The listing builds one solid part. Answer for the finished solid, in the listing's coordinates (mm). A direction names the side the tool comes from. Give positions to 0.01 mm unless a question says otherwise; leave off trailing zeros. Loops run counter-clockwise (first coordinate to the right, second up) from the corner with the lowest first, then second, coordinate; pieces in that order, holes last. Notation, with made-up numbers: M 61.5,-17 L 99.5,-17 A32 ccw 99.5,9 Z; hole C -21,-26 d5. An arc over 180 degrees is marked long. Use one line per item in the form item = value. Start each with the question number.
1. Each of these flat-tipped pins is pushed along its axis until it touches: pin 1 Ø4 at (x, y) = (7.5, 3) entering from +Z; pin 2 Ø1 at (y, z) = (-1, 8) entering from -X; pin 3 Ø3 at (y, z) = (-3.96, 2.69) entering from -X. Where does it stop, or does it pass through?
2. Straight lines are drawn through the part: line 1 (X direction, y = 5.75, z = 1.5); line 2 (X direction, y = -5.5, z = 1); line 3 (Z direction, x = 0.25, y = -2). For each, find the intervals that lie inside material, in ascending order. Write a range as from..to.
3. For faces 1 (the face through (4.2, 2.7, 7.1)), 2 (the face through (-8, 6.636, 5)), 3 (the face through (-4.065, 2.57, 7.071)), 4 (the face through (-8, -1.364, 5)), 5 (the face through (8, -1.364, 5)), determine the directions among +Z, -Z, +X, -X, +Y, -Y from which every point of the face is accessible in a straight line to the end or side of a thin tool.
4. The part is cut by section A-A (y = -3.5). Write down the section's boundary in (x, z), and give its area (3 significant figures).
5. The mould has two halves that part along Y. Classify faces 6 (the face through (0.11, -7.364, 7.15)), 7 (the face through (6.87, -4, 3.69)), 8 (the face through (8, 6.636, 5)), 9 (the face through (-6, 3, 6.5)): released by +Y, released by -Y, zero draft, split by the parting line, or undercut.
6. The part is cut by section B-B (y = -0.75). Write down the section's boundary in (x, z).
from build123d import *

# Parameters (mm, degrees)
CROQUIS2_R                 = 2
SALIENTE_EXTRUIR1_DEPTH    = 6.5
SALIENTE_EXTRUIR1_2_DEPTH  = 6.5
SALIENTE_EXTRUIR2_DEPTH    = 15
CORTAR_EXTRUIR3_START      = -7
CROQUIS7_R                 = 2
CORTAR_EXTRUIR3_DEPTH      = 7
CORTAR_EXTRUIR5_START      = -7.364158067
CORTAR_EXTRUIR5_DEPTH      = 6
CORTAR_EXTRUIR5_START_2    = 6.635841933
CORTAR_EXTRUIR5_2_DEPTH    = 1
CROQUIS13_R                = 4.868357384
CORTAR_EXTRUIR6_DEPTH      = 4
CHAFL_N1_SIZE              = 1
CORTAR_EXTRUIR7_REACH      = 26.966
CORTAR_EXTRUIR7_END_RADIUS = 6
CROQUIS14_R                = 1


# Read off the part's stored shape, not the designer's step: Cortar-Extruir5
with BuildPart() as part:
    # Croquis2 → Saliente-Extruir1 (new body)
    with BuildSketch(Plane.XY):
        with BuildLine():
            ThreePointArc((-8.933187638, -1.364158067), (-12.933187638, 2.635841933), (-8.933187638, 6.635841933))
            Line((-8.933187638, 6.635841933), (-8.933187638, 7.635841933))
            Line((-8.933187638, 7.635841933), (-5.933187638, 7.635841933))
            Line((-5.933187638, 7.635841933), (-5.933187638, -7.364158067))
            Line((-5.933187638, -7.364158067), (-8.933187638, -7.364158067))
            Line((-8.933187638, -7.364158067), (-8.933187638, -1.364158067))
        make_face()
        with Locations(Location((-8.933187638, 2.635841933, 0), (0, 0, 180))):
            Circle(CROQUIS2_R, mode=Mode.SUBTRACT)
    extrude(amount=SALIENTE_EXTRUIR1_DEPTH)



with BuildPart() as body_2:
    # Croquis2 → Saliente-Extruir1 2 (new body)
    with BuildSketch(Plane.XY):
        with BuildLine():
            Line((9.066812362, -1.364158067), (9.066812362, -7.364158067))
            Line((9.066812362, -7.364158067), (6.066812362, -7.364158067))
            Line((6.066812362, -7.364158067), (6.066812362, 7.635841933))
            Line((6.066812362, 7.635841933), (9.066812362, 7.635841933))
            Line((9.066812362, 7.635841933), (9.066812362, 6.635841933))
            ThreePointArc((9.066812362, 6.635841933), (13.066812362, 2.635841933), (9.066812362, -1.364158067))
        make_face()
        with Locations(Location((9.066812362, 2.635841933, 0), (0, 0, 180))):
            Circle(CROQUIS2_R, mode=Mode.SUBTRACT)
    extrude(amount=SALIENTE_EXTRUIR1_2_DEPTH)


with BuildPart() as part_1:
    add(part.part)

    add(body_2.part)  # Saliente-Extruir2 merges body 2
    # Croquis3 → Saliente-Extruir2 (add, through all)
    with BuildSketch(Plane.XZ.offset(7.364158067)):
        with BuildLine():
            Line((-8.933187638, 0), (-5.933187638, 0))
            ThreePointArc((-5.933187638, 0), (0.066812362, 6), (6.066812362, 0))
            Line((6.066812362, 0), (9.066812362, 0))
            ThreePointArc((9.066812362, 0), (0.066812362, 9), (-8.933187638, 0))
        make_face()
    extrude(amount=-SALIENTE_EXTRUIR2_DEPTH)

    # Croquis7 → Cortar-Extruir3 (cut)
    with BuildSketch(Plane.XY.offset(6.5).offset(CORTAR_EXTRUIR3_START)):
        with Locations(Location((9.066812362, 2.635841933, 0), (0, 0, 180))):
            Circle(CROQUIS7_R)
        with Locations(Location((-8.933187638, 2.635841933, 0), (0, 0, 180))):
            Circle(CROQUIS7_R)
    extrude(amount=CORTAR_EXTRUIR3_DEPTH, mode=Mode.SUBTRACT)

    # Cortar-Extruir5 outline → Cortar-Extruir5 (cut)
    with BuildSketch(Plane(origin=(0, 0, 0), x_dir=(1, 0, 0), z_dir=(0, 1, 0)).offset(CORTAR_EXTRUIR5_START)):
        with BuildLine():
            Line((9.066812362, -6.5), (9.066812362, 0))
            ThreePointArc((9.066812362, 0), (8.344026513, -3.53379766), (6.291762161, -6.5))
            Line((6.291762161, -6.5), (9.066812362, -6.5))
        make_face()
        with BuildLine():
            Line((-8.933187638, -6.5), (-6.158137437, -6.5))
            ThreePointArc((-6.158137437, -6.5), (-8.210401789, -3.53379766), (-8.933187638, 0))
            Line((-8.933187638, 0), (-8.933187638, -6.5))
        make_face()
    extrude(amount=CORTAR_EXTRUIR5_DEPTH, mode=Mode.SUBTRACT)

    # Cortar-Extruir5 2 outline → Cortar-Extruir5 2 (cut)
    with BuildSketch(Plane(origin=(0, 0, 0), x_dir=(1, 0, 0), z_dir=(0, 1, 0)).offset(CORTAR_EXTRUIR5_START_2)):
        with BuildLine():
            Line((9.066812362, -6.5), (9.066812362, 0))
            ThreePointArc((9.066812362, 0), (8.344026513, -3.53379766), (6.291762161, -6.5))
            Line((6.291762161, -6.5), (9.066812362, -6.5))
        make_face()
        with BuildLine():
            Line((-8.933187638, -6.5), (-6.158137437, -6.5))
            ThreePointArc((-6.158137437, -6.5), (-8.210401789, -3.53379766), (-8.933187638, 0))
            Line((-8.933187638, 0), (-8.933187638, -6.5))
        make_face()
    extrude(amount=CORTAR_EXTRUIR5_2_DEPTH, mode=Mode.SUBTRACT)

    # Croquis13 → Cortar-Extruir6 (cut)
    with BuildSketch(Plane.XY.offset(6.5)):
        with Locations((9.066812362, 2.635841933)):
            Circle(CROQUIS13_R)
        with Locations((-8.933187638, 2.635841933)):
            Circle(CROQUIS13_R)
    extrude(amount=CORTAR_EXTRUIR6_DEPTH, mode=Mode.SUBTRACT)

    # Chaflán1
    chafl_n1_edges = [part_1.edges().sort_by_distance(p)[0] for p in [
        (0.066812362, 7.635841933, 6),
        (0.066812362, -7.364158067, 6),
    ]]
    chamfer(chafl_n1_edges, length=CHAFL_N1_SIZE)

    # Cortar-Extruir7: up to this cylinder (the profile starts outside it)
    cortar_extruir7_end = Plane(origin=(0.066812362, -3.95674, 0), z_dir=(0, -1, 0)) * Cylinder(CORTAR_EXTRUIR7_END_RADIUS, 66.932, mode=Mode.PRIVATE)
    # Croquis14 → Cortar-Extruir7 (cut, up to the surface)
    with BuildSketch(Plane(origin=(9.066812362, 0, 0), x_dir=(0, -1, 0), z_dir=(-1, 0, 0)), mode=Mode.PRIVATE) as cortar_extruir7_sk1:
        with Locations(Location((3.956739881, 2.692300291, 0), (0, 0, 270))):
            Circle(CROQUIS14_R)
    cortar_extruir7_tool1 = extrude(cortar_extruir7_sk1.sketch, amount=CORTAR_EXTRUIR7_REACH, mode=Mode.PRIVATE) - cortar_extruir7_end
    add(cortar_extruir7_tool1.solids().sort_by_distance((9.066812, -3.95674, 2.6923))[0], mode=Mode.SUBTRACT)


solid = part_1.part
Derived:
q1.pin_1 = 6.5
q1.pin_2 = -4.91
q1.pin_3 = -8.85
q2.line_1 = -11.44..-5.74, 5.88..11.58
q2.line_2 = -8.88..-5.85, 5.98..9.01
q2.line_3 = 6..9
q3.face_1 = +Z, +X
q3.face_2 = +Z, -X, +Y
q3.face_3 = +Z, -X
q3.face_4 = +Z, -X, -Y
q3.face_5 = +Z, +X, -Y
q4.outline = M -8.93,0 L -5.93,0 A6 cw 4.88,3.58 L 8.32,3.58 A9 ccw Z; M 5.79,1.8 A6 cw 6.07,0 L 9.07,0 A9 ccw 8.88,1.8 Z
q4.area = 64.9 mm2
q5.face_6 = released by -Y
q5.face_7 = undercut
q5.face_8 = released by +Y
q5.face_9 = undercut
q6.outline = M -11.06,0 L -5.93,0 A6 cw 6.07,0 L 11.2,0 L 11.2,6.5 L 5.57,6.5 L 5.57,7.12 A9 ccw -5.44,7.12 L -5.44,6.5 L -11.06,6.5 Z
